Drawing for the job (mm, zero at the part's lowest x, y, z). A direction names the side the tool comes from. Round coordinates to 2 decimals unless told otherwise and drop trailing zeros. Order: outer loops, then holes, each group sorted by start corner. A loop starts at its lowest first (then second) coordinate and runs counter-clockwise, first axis right, second up. Notation, with made-up numbers: (12.5, 1.25) - (18.5, 1.25) arc R29 ccw to (18.5, 22.25) - close; hole circle Ø8 at (-2, -5.75). An arc over 180 degrees is marked (long way). Answer as a JSON object with one key per item and string values.
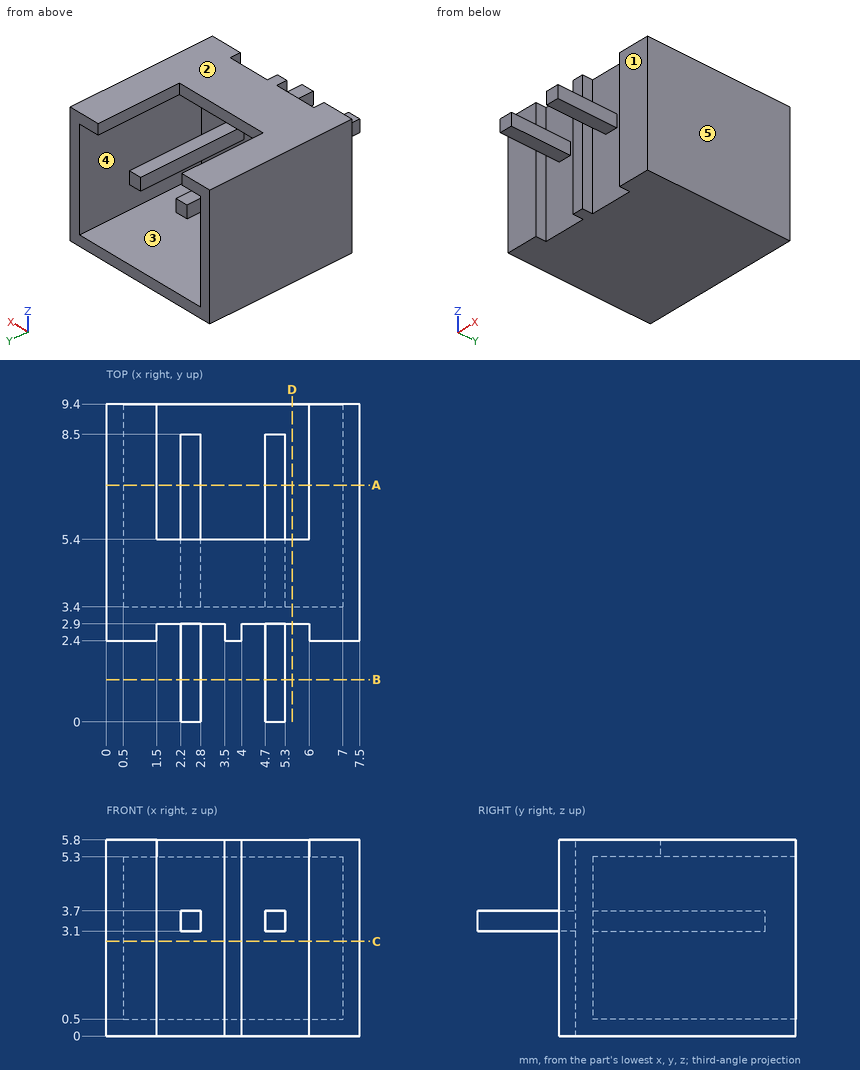
Item 1: Cut at B-B (y = 1.25). Write the cut outline in (x, z).
Taken from the geometry:
{"outline": "(2.2, 3.1) - (2.8, 3.1) - (2.8, 3.7) - (2.2, 3.7) - close; (4.7, 3.1) - (5.3, 3.1) - (5.3, 3.7) - (4.7, 3.7) - close"}
Item 2: Cut at A-A (y = 7). Write the cut outline in (x, z).
Taken from the geometry:
{"outline": "(0, 0) - (7.5, 0) - (7.5, 5.8) - (6, 5.8) - (6, 5.3) - (7, 5.3) - (7, 0.5) - (0.5, 0.5) - (0.5, 5.3) - (1.5, 5.3) - (1.5, 5.8) - (0, 5.8) - close; (2.2, 3.1) - (2.8, 3.1) - (2.8, 3.7) - (2.2, 3.7) - close; (4.7, 3.1) - (5.3, 3.1) - (5.3, 3.7) - (4.7, 3.7) - close"}
Item 3: Tool access for the marked faces 4 and 5: list every direction of +Z, -Z, +X, -X, +Y, -Y with a clear straight run to the whole face (end or side of a thin tool).
Taken from the geometry:
{"face 4": "+Y", "face 5": "+Z, -Z, +X, +Y, -Y"}
Item 4: Cut at C-C (z = 2.8). Write the cut outline in (x, y).
Taken from the geometry:
{"outline": "(0, 2.4) - (1.5, 2.4) - (1.5, 2.9) - (3.5, 2.9) - (3.5, 2.4) - (4, 2.4) - (4, 2.9) - (6, 2.9) - (6, 2.4) - (7.5, 2.4) - (7.5, 9.4) - (7, 9.4) - (7, 3.4) - (0.5, 3.4) - (0.5, 9.4) - (0, 9.4) - close"}
Item 5: Two-plate mould, pull along Z, no slides. Class the marked faces 1, 2 and 3: pulls with the +Z half, pulls with the -Z half, needs draft (parallel to the pull), parting line crosses it, or undercut.
Taken from the geometry:
{"face 1": "needs draft", "face 2": "pulls with the +Z half", "face 3": "undercut"}
Item 6: Drop flat-ended pins along their axis: P1, Ø2, axis at x = 4, y = 8.5, coming from the +Z side; P2, Ø1.2, axis at x = 0.5, z = 2.5, coming from the -Y side; P3, Ø0.5, axis at x = 5, z = 3.5, coming from the +Y side. Give the stop position or say it passes through.
Taken from the geometry:
{"P1": "z = 3.7", "P2": "y = 2.4", "P3": "y = 8.5"}
Item 7: Cut at D-D (x = 5.5). Write the cut outline in (y, z).
Taken from the geometry:
{"outline": "(2.9, 0) - (9.4, 0) - (9.4, 0.5) - (3.4, 0.5) - (3.4, 5.3) - (5.4, 5.3) - (5.4, 5.8) - (2.9, 5.8) - close"}
Item 8: Probe L1, parallel to Z at x = 2.5, y = 5; L2, parallel to X at y = 4, z = 3.4; L3, parallel to Z at x = 1.75, y = 5.25. List the from-to ranges inside material, lowest first. Write a range as from..to.
Taken from the geometry:
{"L1": "0..0.5, 3.1..3.7, 5.3..5.8", "L2": "0..0.5, 2.2..2.8, 4.7..5.3, 7..7.5", "L3": "0..0.5, 5.3..5.8"}
